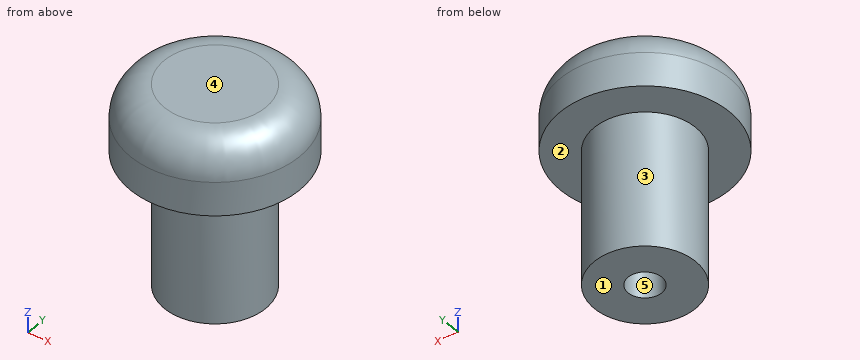
from build123d import *

# Parameters (mm, degrees)
SKETCH1_R           = 2.5
BOSS_EXTRUDE1_DEPTH = 2
SKETCH2_R           = 1.5
BOSS_EXTRUDE2_DEPTH = 4
FILLET2_R           = 1
SKETCH3_R           = 0.5
CUT_EXTRUDE1_DEPTH  = 2


with BuildPart() as part:
    # Sketch1 → Boss-Extrude1 (new body)
    with BuildSketch(Plane.XY):
        Circle(SKETCH1_R)
    extrude(amount=-BOSS_EXTRUDE1_DEPTH)

    # Sketch2 → Boss-Extrude2 (add)
    with BuildSketch(Plane(origin=(0, 0, -2), x_dir=(-1, 0, 0), z_dir=(0, 0, -1))):
        Circle(SKETCH2_R)
    extrude(amount=BOSS_EXTRUDE2_DEPTH)

    # Fillet2
    fillet2_edges = [part.edges().sort_by_distance(p)[0] for p in [
        (-2.5, 0, 0),
    ]]
    fillet(fillet2_edges, radius=FILLET2_R)

    # Sketch3 → Cut-Extrude1 (cut)
    with BuildSketch(Plane(origin=(0, 0, -6), x_dir=(-1, 0, 0), z_dir=(0, 0, -1))):
        Circle(SKETCH3_R)
    extrude(amount=-CUT_EXTRUDE1_DEPTH, mode=Mode.SUBTRACT)


solid = part.part
Work out the finished part from the listing and answer in its coordinate system (mm). Face numbers are marked on the shaded views. A direction names the side the tool comes from. Coordinates: 2 decimals unless noted, no trailing zeros. Write each loop counter-clockwise with the first axis right and the second up, starting at its lowest first coordinate (ties: lowest second). Pieces come first, ordered by that corner, then holes. Notation, with made-up numbers: M 63,-12 L 86,-12 A21 ccw 86,-3 Z; hole C 57,38.5 d7. An arc over 180 degrees is marked long. Answer as CSV lines item,"result". Start each with the question number.
Item 1: A tool of negligible diameter and unlimited length cuts with its end or side. For the marked faces 1 and 2, from which of +Z, -Z, +X, -X, +Y, -Y can it reach the whole face along a straight path? Write none if from no direction.
Item 2: Flat-ended cylindrical pins translate along their axes: P1, Ø1, axis at x = 1.5, z = -1.5, coming from the +Y side; P2, Ø1.5, axis at x = 1.5, z = -3, coming from the +Y side. Find the tip coordinate at first contact, or state that the pin passes through.
Item 3: Determine the mould class of the marked faces 3, 4 and 5 for opening direction Y: released by +Y, released by -Y, zero draft, split by the parting line, or undercut.
Item 4: Section A-A on y = 0 is taken. Write down the section's boundary in (x, z).
Item 5: Section C-C on z = -2.55 is taken. Write down the section's boundary in (x, y).
Item 6: Consider L1, parallel to Y at x = 0, z = -5.25; L2, parallel to Z at x = 1, y = 1.2; L3, parallel to Y at x = 0.6, z = -5. Determine where each line is inside the solid, lowest interval first.
Item 7: Section D-D on z = -4.45 is taken. Write down the section's boundary in (x, y).
Checks:
1,face 1,"-Z, +X, -X, +Y, -Y"
1,face 2,"-Z"
2,P1,"stops at y = 2.29"
2,P2,"stops at y = 1.3"
3,face 3,"split by the parting line"
3,face 4,"zero draft"
3,face 5,"undercut"
4,outline,"M -2.5,-2 L -1.5,-2 L -1.5,-6 L -0.5,-6 L -0.5,-4 L 0.5,-4 L 0.5,-6 L 1.5,-6 L 1.5,-2 L 2.5,-2 L 2.5,-1 A1 ccw 1.5,0 L -1.5,0 A1 ccw -2.5,-1 Z"
5,outline,"C 0,0 d3"
6,L1,"y = -1.5 to -0.5, 0.5 to 1.5"
6,L2,"z = -2 to 0"
6,L3,"y = -1.37 to 1.37"
7,outline,"C 0,0 d3; hole C 0,0 d1"
